from build123d import *

# Parameters (mm, degrees)
SKETCH1_W           = 330
SKETCH1_H           = 450
BOSS_EXTRUDE1_DEPTH = 500
SKETCH2_W           = 200
SKETCH2_H           = 350
CUT_EXTRUDE1_DEPTH  = 100
BOSS_EXTRUDE2_DEPTH = 100
SKETCH4_W           = 200
SKETCH4_H           = 20
BOSS_EXTRUDE3_DEPTH = 200
SKETCH5_R           = 58.984993577
CUT_EXTRUDE2_DEPTH  = 50
FILLET1_R           = 10
SKETCH6_W           = 108.793875533
SKETCH6_H           = 71.48855694
BOSS_EXTRUDE4_DEPTH = 50
FILLET2_R           = 5
FILLET3_R           = 10
SKETCH7_W           = 6.282051282
SKETCH7_H           = 70
CUT_EXTRUDE3_DEPTH  = 20


with BuildPart() as part:
    # Sketch1 → Boss-Extrude1 (new body)
    with BuildSketch(Plane(origin=(0, 0, 0), x_dir=(1, 0, 0), z_dir=(0, 1, 0))):
        Rectangle(SKETCH1_W, SKETCH1_H)
    extrude(amount=BOSS_EXTRUDE1_DEPTH)

    # Sketch2 → Cut-Extrude1 (cut)
    with BuildSketch(Plane.XY.offset(225)):
        with Locations((0, 175)):
            Rectangle(SKETCH2_W, SKETCH2_H)
    extrude(amount=-CUT_EXTRUDE1_DEPTH, mode=Mode.SUBTRACT)

    # Sketch3 → Boss-Extrude2 (add)
    with BuildSketch(Plane.XZ.offset(-350)):
        with BuildLine():
            Line((100, 225), (-100, 225))
            ThreePointArc((-100, 225), (0, 284.9775435), (100, 225))
        make_face()
    extrude(amount=-BOSS_EXTRUDE2_DEPTH)

    # Sketch4 → Boss-Extrude3 (add)
    with BuildSketch(Plane.XY.offset(125)):
        with Locations((0, 10)):
            Rectangle(SKETCH4_W, SKETCH4_H)
    extrude(amount=BOSS_EXTRUDE3_DEPTH)

    # Sketch5 → Cut-Extrude2 (cut)
    with BuildSketch(Plane.XZ.offset(-350)):
        with Locations((0, 203.171289973)):
            Circle(SKETCH5_R)
    extrude(amount=-CUT_EXTRUDE2_DEPTH, mode=Mode.SUBTRACT)

    # Fillet1
    fillet1_edges = [part.edges().sort_by_distance(p)[0] for p in [
        (165, 250, 225),
        (-165, 250, 225),
        (-165, 250, -225),
        (165, 250, -225),
    ]]
    fillet(fillet1_edges, radius=FILLET1_R)

    # Sketch6 → Boss-Extrude4 (add)
    with BuildSketch(Plane(origin=(0, 0, -225), x_dir=(-1, 0, 0), z_dir=(0, 0, -1))):
        with Locations((-86.447180312, 35.74427847)):
            Rectangle(SKETCH6_W, SKETCH6_H)
    extrude(amount=BOSS_EXTRUDE4_DEPTH)

    # Fillet2
    fillet2_edges = [part.edges().sort_by_distance(p)[0] for p in [
        (140.844118078, 71.48855694, -250),
        (140.844118078, 0, -250),
        (32.050242545, 0, -250),
        (32.050242545, 71.48855694, -250),
    ]]
    fillet(fillet2_edges, radius=FILLET2_R)

    # Fillet3
    fillet3_edges = [part.edges().sort_by_distance(p)[0] for p in [
        (-100, 10, 325),
        (100, 10, 325),
    ]]
    fillet(fillet3_edges, radius=FILLET3_R)

    # Sketch7 → Cut-Extrude3 (cut)
    with BuildSketch(Plane(origin=(0, 500, 0), x_dir=(1, 0, 0), z_dir=(0, 1, 0))):
        with Locations((-65.512820513, 35)):
            Rectangle(SKETCH7_W, SKETCH7_H)
        with BuildLine():
            Line((20.192307692, 57.155448718), (14.695512821, 52.948717949))
            add(Edge.make_bspline(
                [(14.695512821, 52.948717949), (14.303395053, 53.416037345), (13.524446117, 54.34437566), (12.271262066, 55.647966549), (10.965229208, 56.869271778), (9.606846784, 58.01410937), (8.171664394, 59.042444685), (6.694448421, 60.007866744), (5.150487517, 60.873221503), (3.015452824, 61.922481225), (0.222495858, 63.017404325), (-3.293400923, 63.935468951), (-6.963622893, 64.519892465), (-9.467574885, 64.583189294), (-10.741185897, 64.615384615)],
                knots=[0, 0, 0, 0, 0.757959112, 1.505699292, 2.245454638, 2.979532153, 3.711538275, 4.438200793, 5.171680507, 5.909471876, 7.393775596, 8.890124382, 10.418191784, 12, 12, 12, 12], degree=3))
            add(Edge.make_bspline(
                [(-10.741185897, 64.615384615), (-11.442851884, 64.607305365), (-12.839671736, 64.591221848), (-14.912641206, 64.379039344), (-16.946902228, 64.080815143), (-18.941131553, 63.638308678), (-20.892790723, 63.078856297), (-22.814638765, 62.410348018), (-24.678850761, 61.583251221), (-26.511215525, 60.669086022), (-28.266799745, 59.636537127), (-29.9279007, 58.51027009), (-31.488460059, 57.302888161), (-32.949712302, 56.009866033), (-34.313151268, 54.637026824), (-35.568897484, 53.169739992), (-36.71260569, 51.612696522), (-37.766946191, 49.98642837), (-38.711200858, 48.295672538), (-39.501798446, 46.534171129), (-40.20190089, 44.732089068), (-40.755885743, 42.869065852), (-41.194376079, 40.958210535), (-41.496929345, 38.994394776), (-41.706698769, 36.981721184), (-41.722702307, 35.617534932), (-41.730769231, 34.929887821)],
                knots=[0, 0, 0, 0, 1.054917814, 2.100044995, 3.131103042, 4.146048494, 5.169673617, 6.183595914, 7.203665975, 8.234915748, 9.262203917, 10.264457458, 11.251630812, 12.227803204, 13.197192746, 14.159520551, 15.12972552, 16.100847026, 17.073214652, 18.039054194, 19.002613845, 19.979014051, 20.95965708, 21.949030935, 22.966165397, 24, 24, 24, 24], degree=3))
            add(Edge.make_bspline(
                [(-41.730769231, 34.929887821), (-41.70553285, 33.895261422), (-41.655984565, 31.863909725), (-41.215017883, 28.888497514), (-40.544916057, 26.038084039), (-39.540604519, 23.330487192), (-38.302223507, 20.732320031), (-36.737411277, 18.287542963), (-34.92508053, 15.959211673), (-32.839592141, 13.802352718), (-30.551475821, 11.832078212), (-28.096517589, 10.097066582), (-25.480831833, 8.650768932), (-22.73329923, 7.447250002), (-19.832776951, 6.522115449), (-16.784480903, 5.870832979), (-13.595040998, 5.445989368), (-11.415653, 5.405315607), (-10.306490385, 5.384615385)],
                knots=[0, 0, 0, 0, 1.029171465, 2.020641659, 2.987623507, 3.938342917, 4.889210282, 5.84687017, 6.821220943, 7.821438502, 8.827599549, 9.822697543, 10.807740252, 11.797342354, 12.80366471, 13.83203677, 14.896651826, 16, 16, 16, 16], degree=3))
            add(Edge.make_bspline(
                [(-10.306490385, 5.384615385), (-9.084436605, 5.41839098), (-6.679142426, 5.48486943), (-3.1517819, 6.048054413), (0.224933413, 6.96121277), (3.451185144, 8.239171216), (6.517878068, 9.900476974), (9.429811274, 11.914434522), (12.189442684, 14.300201177), (13.848868329, 16.121863743), (14.695512821, 17.051282051)],
                knots=[0, 0, 0, 0, 1.028121516, 2.023589091, 2.998037872, 3.967518031, 4.937445131, 5.927275754, 6.942489185, 8, 8, 8, 8], degree=3))
            Line((14.695512821, 17.051282051), (20.192307692, 12.88661859))
            add(Edge.make_bspline(
                [(20.192307692, 12.88661859), (19.749945495, 12.315849551), (18.867339989, 11.177045426), (17.43817965, 9.571611231), (15.932633702, 8.061530521), (14.339519502, 6.658978097), (12.67716367, 5.335888785), (10.915717423, 4.129852159), (9.078336773, 3.024034474), (7.171247195, 2.011495983), (5.196474939, 1.113151043), (3.15638624, 0.344075687), (1.05977473, -0.318422104), (-1.093455438, -0.863460838), (-3.307770575, -1.288882516), (-5.575180057, -1.573276013), (-7.900577561, -1.768114301), (-9.469405984, -1.785872618), (-10.264423077, -1.794871795)],
                knots=[0, 0, 0, 0, 0.986787822, 1.968848986, 2.935600012, 3.899624008, 4.868462664, 5.837806735, 6.815139263, 7.798259679, 8.787526145, 9.778297419, 10.776456485, 11.791383307, 12.812564526, 13.85620153, 14.913611965, 16, 16, 16, 16], degree=3))
            add(Edge.make_bspline(
                [(-10.264423077, -1.794871795), (-11.017296418, -1.789631944), (-12.50601022, -1.779270787), (-14.703985252, -1.611427439), (-16.843776868, -1.382432701), (-18.919269386, -1.037630079), (-20.941788887, -0.630743278), (-22.893000576, -0.085318146), (-24.792104784, 0.525665186), (-26.631471597, 1.243764921), (-28.412665593, 2.054088572), (-30.129941821, 2.96991975), (-31.782510469, 3.983557043), (-33.386618886, 5.072657252), (-34.918570559, 6.272203289), (-36.391641066, 7.565535979), (-37.814090591, 8.948296194), (-38.694144291, 9.945393261), (-39.13661859, 10.446714744)],
                knots=[0, 0, 0, 0, 1.114604814, 2.203992996, 3.262667896, 4.300477797, 5.318619304, 6.316056647, 7.298880507, 8.271930387, 9.238335007, 10.195173496, 11.151986948, 12.108099108, 13.064862484, 14.031167946, 15.010108607, 16, 16, 16, 16], degree=3))
            add(Edge.make_bspline(
                [(-39.13661859, 10.446714744), (-39.84533146, 11.317538522), (-41.254200996, 13.04867273), (-43.056714667, 15.854392355), (-44.599665772, 18.783756533), (-45.847184187, 21.852155108), (-46.82243885, 25.052702853), (-47.498062752, 28.387013141), (-47.937094841, 31.851971985), (-47.987300617, 34.208707759), (-48.012820513, 35.406650641)],
                knots=[0, 0, 0, 0, 0.994628077, 1.977248131, 2.950237994, 3.925870899, 4.908910175, 5.911660606, 6.938484602, 8, 8, 8, 8], degree=3))
            add(Edge.make_bspline(
                [(-48.012820513, 35.406650641), (-47.981716642, 36.665759712), (-47.920521717, 39.142978203), (-47.400605808, 42.778457269), (-46.564229884, 46.261485246), (-45.376292112, 49.585560138), (-43.870185086, 52.768165742), (-42.009652809, 55.784989839), (-39.816309965, 58.655325832), (-37.307358611, 61.335620858), (-34.556011905, 63.786407911), (-31.609635627, 65.942531986), (-28.473996688, 67.736882306), (-25.183639654, 69.236805554), (-21.713926023, 70.389694817), (-18.07225864, 71.196758551), (-14.265480345, 71.699100877), (-11.668231832, 71.762605035), (-10.348557692, 71.794871795)],
                knots=[0, 0, 0, 0, 1.032925535, 2.032216505, 3.007276963, 3.968222605, 4.92396291, 5.891752235, 6.871517503, 7.883894988, 8.900124299, 9.891468569, 10.874487609, 11.85992873, 12.854644235, 13.869047385, 14.917252991, 16, 16, 16, 16], degree=3))
            add(Edge.make_bspline(
                [(-10.348557692, 71.794871795), (-9.544268253, 71.785229031), (-7.952258307, 71.766142151), (-5.597205259, 71.580019309), (-3.30435872, 71.269747184), (-1.07213908, 70.847425788), (1.110313244, 70.323279359), (3.226318062, 69.640473392), (5.288291799, 68.859742766), (7.283229963, 67.960573447), (9.201560966, 66.951238619), (11.042687336, 65.842926148), (12.79198451, 64.637010038), (14.461761479, 63.34374653), (16.0240857, 61.935775344), (17.523315271, 60.451823425), (18.908536834, 58.849146941), (19.763600734, 57.721048263), (20.192307692, 57.155448718)],
                knots=[0, 0, 0, 0, 1.096760587, 2.17092713, 3.219439832, 4.250915756, 5.268269357, 6.278326846, 7.281116186, 8.274029601, 9.260640565, 10.235837813, 11.203064059, 12.156899882, 13.114053108, 14.069676657, 15.032185724, 16, 16, 16, 16], degree=3))
        make_face()
        Polygon((34.551282051, 70), (74.038461538, 70), (74.038461538, 62.820512821), (40.833333333, 62.820512821), (40.833333333, 41.282051282), (74.038461538, 41.282051282), (74.038461538, 34.102564103), (40.833333333, 34.102564103), (40.833333333, 7.179487179), (74.038461538, 7.179487179), (74.038461538, 0), (34.551282051, 0), align=None)
    extrude(amount=-CUT_EXTRUDE3_DEPTH, mode=Mode.SUBTRACT)


solid = part.part
Here's how the part is built. I have some questions about the finished solid (model axes, mm). A direction names the side the tool comes from. Coordinates: 2 decimals unless noted, no trailing zeros. Order: outer loops, then holes, each group sorted by start corner. A loop starts at its lowest first (then second) coordinate and runs counter-clockwise, first axis right, second up. Notation, with made-up numbers: (5, 80) -> (63, 80) arc R24 cw to (63, 102) -> close; hole circle Ø3 at (47, -2). An arc over 180 degrees is marked (long way). Answer in a Markdown table with one row per item.
(1) I want a section at C-C on x = 108. List the corners of the cut face in (y, z) for me.
Answer key:
| item | result |
|---|---|
| outline | (0, -275) -> (71.49, -275) -> (71.49, -225) -> (500, -225) -> (500, 225) -> (0, 225) -> close |
(2) Thinking about a two-plate mould opening in X: for faces 5 (the face through (-1.715, 399.3, 284.965)), 6 (the face through (140.844, 35, -250)), 7 (the face through (87, 71.489, -250)), 8 (the face through (57, 490, -41.282)), which applies, +X half, -X half, draft (parallel to the pull), parting line (faces both ways), or undercut?
Answer key:
| item | result |
|---|---|
| face 5 | parting line |
| face 6 | +X half |
| face 7 | draft |
| face 8 | undercut |
(3) I want a section at A-A on y = 89.5. List the corners of the cut face in (x, z) for me, then the cut area to 3 significant figures.
Answer key:
| item | result |
|---|---|
| outline | (-165, -215) arc R10 ccw to (-155, -225) -> (155, -225) arc R10 ccw to (165, -215) -> (165, 215) arc R10 ccw to (155, 225) -> (100, 225) -> (100, 125) -> (-100, 125) -> (-100, 225) -> (-155, 225) arc R10 ccw to (-165, 215) -> close |
| area | 128,000 mm^2 |
(4) I want a section at B-B on z = 246. List the corners of the cut face in (x, y) for me, then the cut area to 3 significant figures.
Answer key:
| item | result |
|---|---|
| outline | (-100, 0) -> (100, 0) -> (100, 20) -> (-100, 20) -> close; (-85.54, 350) -> (-40.56, 350) -> (-40.56, 400) -> (40.56, 400) -> (40.56, 350) -> (85.54, 350) -> (85.54, 450) -> (-85.54, 450) -> close |
| area | 17,100 mm^2 |
(5) On a 3-axis mill with a long thin cutter (end or side, diameter ignored), from which of +Z, -Z, +X, -X, +Y, -Y can I reach the whole of each face in a straight line? I mean faces 1 (the face through (-1, 187, 125)), 2 (the face through (55, 490, 0)), 3 (the face through (-12.79, 374.65, 145.59)), 4 (the face through (87, 36, -275)). Say none if no direction works.
Answer key:
| item | result |
|---|---|
| face 1 | +Z |
| face 2 | +Y |
| face 3 | none |
| face 4 | -Z, +X, -X, +Y, -Y |
(6) Please list where these lines run through material, in increasing order: probe 1 along Z at (x, y) = (0, 373); probe 2 along X at (y, z) = (194.5, 178.5); probe 3 along Y at (x, z) = (-55, 234).
Answer key:
| item | result |
|---|---|
| probe 1 | -225 to 144.19, 262.16 to 284.98 |
| probe 2 | -165 to -100, 100 to 165 |
| probe 3 | 0 to 20, 350 to 450 |
(7) Will these pins go through, and if not, where does the flat tip stop? pin 1 Ø10 at (x, y) = (58.5, 486.5) entering from -Z; pin 2 Ø15 at (y, z) = (48, -250) entering from +X; pin 3 Ø7 at (x, y) = (-66, 489.5) entering from +Z.
Answer key:
| item | result |
|---|---|
| pin 1 | z = -225 |
| pin 2 | x = 140.84 |
| pin 3 | z = 225 |
